```python
from build123d import *

# Parameters (mm, degrees)
SKETCH1_W               = 673.1
SKETCH1_H               = 204.6732
BOSS_EXTRUDE1_DEPTH     = 9.525
SKETCH2_R               = 9.584587104
CUT_EXTRUDE1_DEPTH      = 1
CUT_EXTRUDE1_DEPTH_BACK = 20.05
SKETCH4_W               = 673.1
SKETCH4_H               = 4.699
CUT_EXTRUDE2_DEPTH      = 10.16
CUT_EXTRUDE5_DEPTH      = 7.9375


with BuildPart() as part:
    # Sketch1 → Boss-Extrude1 (new body, symmetric)
    with BuildSketch(Plane(origin=(0, 0, 0), x_dir=(1, 0, 0), z_dir=(0, 1, 0))):
        Rectangle(SKETCH1_W, SKETCH1_H)
    extrude(amount=BOSS_EXTRUDE1_DEPTH, both=True)

    # Sketch2 → Cut-Extrude1 (cut, two sides)
    with BuildSketch(Plane(origin=(0, 9.525, 0), x_dir=(1, 0, 0), z_dir=(0, 1, 0))) as cut_extrude1_sk:
        with Locations((-304.8, 76.930371018)):
            Circle(SKETCH2_R)
        with Locations((-237.0709, 76.930371018)):
            Circle(SKETCH2_R)
        with Locations((-169.3418, 76.930371018)):
            Circle(SKETCH2_R)
        with Locations((-101.6127, 76.930371018)):
            Circle(SKETCH2_R)
        with Locations((-33.8836, 76.930371018)):
            Circle(SKETCH2_R)
        with Locations((33.8455, 76.930371018)):
            Circle(SKETCH2_R)
        with Locations((101.5746, 76.930371018)):
            Circle(SKETCH2_R)
        with Locations((169.3037, 76.930371018)):
            Circle(SKETCH2_R)
        with Locations((237.0328, 76.930371018)):
            Circle(SKETCH2_R)
        with Locations((304.7619, 76.930371018)):
            Circle(SKETCH2_R)
    extrude(amount=CUT_EXTRUDE1_DEPTH, mode=Mode.SUBTRACT)
    extrude(cut_extrude1_sk.sketch, amount=-CUT_EXTRUDE1_DEPTH_BACK, mode=Mode.SUBTRACT)

    # Sketch4 → Cut-Extrude2 (cut)
    with BuildSketch(Plane.XZ.offset(9.525)):
        with Locations((0, 93.6860458)):
            Rectangle(SKETCH4_W, SKETCH4_H)
    extrude(amount=-CUT_EXTRUDE2_DEPTH, mode=Mode.SUBTRACT)

    # Sketch7 → Cut-Extrude5 (cut)
    with BuildSketch(Plane.XZ.offset(9.525)):
        with BuildLine():
            Line((-323.05625, -26.291096465), (323.05625, -26.291096465))
            ThreePointArc((323.05625, -26.291096465), (331.05725, -34.292096465), (323.05625, -42.293096465))
            Line((323.05625, -42.293096465), (-323.05625, -42.293096465))
            ThreePointArc((-323.05625, -42.293096465), (-331.05725, -34.292096465), (-323.05625, -26.291096465))
        make_face()
    extrude(amount=-CUT_EXTRUDE5_DEPTH, mode=Mode.SUBTRACT)


solid = part.part
```
Check sheet for the modelled part. Datum: model origin and axes. Units: mm. Coordinates: 2 decimals unless noted, no trailing zeros. Order: outer loops, then holes, each group sorted by start corner. A loop starts at its lowest first (then second) coordinate and runs counter-clockwise, first axis right, second up. Notation, with made-up numbers: M 32,37.25 L 76,37.25 A26 cw 76,75.25 Z; hole C -30.75,-12 d8. An arc over 180 degrees is marked long. Write each question's results on one line, items separated by ' | '. Start each with the question number.
1. Mould release check, pull along Z, two halves, no side actions. Record for faces 1 (the face through (-5, 0, -102.337)), 2 (the face through (-5, 0, 102.337)), 3 (the face through (5, -1.588, -34)), 4 (the face through (-336.55, 0, 1)): +Z half, -Z half, draft (parallel to the pull), parting line (faces both ways), or undercut.
2. Cross-section at A-A on y = -5.25. State how many separate pieces and enclosed holes the cut face has, and give its area (3 significant figures).
3. Cross-section at B-B on x = -304.8. Record the cut outline in (y, z) (1 decimal).
4. Material ranges on probe 1 along Z at (x, y) = (-262, -5.75); probe 2 along Z at (x, y) = (129, -1.5); probe 3 along Z at (x, y) = (232.5, -8), recorded low to high.
5. Go/stop test with flat-tipped pins: P1, Ø1.4, axis at x = -81, z = 93, coming from the -Y side (3 decimals); P2, Ø15.5, axis at x = 237.03, z = -76.93, coming from the +Y side. Record where each tip stops, or that it passes through.
Checks:
1) face 1: -Z half | face 2: +Z half | face 3: undercut | face 4: draft
2) separate pieces: 2 | enclosed holes: 11 | area: 121,000 mm²
3) outline: M -9.5,-102.3 L 9.5,-102.3 L 9.5,-86.5 L -9.5,-86.5 Z; M -9.5,-67.3 L 9.5,-67.3 L 9.5,102.3 L -9.5,102.3 L -9.5,96 L 0.6,96 L 0.6,91.3 L -9.5,91.3 L -9.5,-26.3 L -1.6,-26.3 L -1.6,-42.3 L -9.5,-42.3 Z
4) probe 1: z = -102.34 to -42.29, -26.29 to 91.34, 96.04 to 102.34 | probe 2: z = -102.34 to 91.34, 96.04 to 102.34 | probe 3: z = -102.34 to -85.38, -68.49 to -42.29, -26.29 to 91.34, 96.04 to 102.34
5) P1: stops at y = 0.635 | P2: passes through
